```python
from build123d import *

# Parameters (mm, degrees)
F0_W      = 95.741764
F0_H      = 56.171074
F1_DEPTH  = 76.2
F1_FACE_W = 95.741764
F1_FACE_H = 56.171074
F2_DEPTH  = 25.4
F3_W      = 43.624266
F3_H      = 23.742414
F4_DEPTH  = 25.4


with BuildPart() as f1:
    # F0 (on Top) → F1 (new body)
    with BuildSketch(Plane.XY):
        Rectangle(F0_W, F0_H)
    extrude(amount=F1_DEPTH)

    # F1_face (on face) → F2 (join)
    with BuildSketch(Plane.XY.offset(76.2)):
        Rectangle(F1_FACE_W, F1_FACE_H)
    extrude(amount=F2_DEPTH)

    # F3 (on face) → F4 (cut)
    with BuildSketch(Plane.XY.offset(101.6)):
        Rectangle(F3_W, F3_H)
    extrude(amount=-F4_DEPTH, mode=Mode.SUBTRACT)


solid = f1.part
```
Model file for the job. Use its own axes, mm. A direction names the side the tool comes from. Coordinates: 2 decimals unless noted, no trailing zeros. Write each loop counter-clockwise with the first axis right and the second up, starting at its lowest first coordinate (ties: lowest second). Pieces come first, ordered by that corner, then holes. Notation, with made-up numbers: (3.25, 7) - (16.25, 7) arc R15 cw to (16.25, 20) - close; hole circle Ø1 at (25.5, 64.25). An arc over 180 degrees is marked (long way). One line per question, with ' | ' between items. Start each with the question number.
Q1. Pull direction X, two halves, no side cores. Call faces 3 (the face through (-47.871, 0, 50)), 4 (the face through (0, 11.871, 89)), 5 (the face through (0, 0, 76.2)), 6 (the face through (-1, 0, 0)): pulls with the +X half, pulls with the -X half, needs draft (parallel to the pull), parting line crosses it, or undercut.
Q2. Cut at B-B, the plane x = -10. List the corners of the cut face in (y, z), then the cut area to 3 significant figures.
Q3. Pin check, flat tip, straight feed: pin 1 (12 mm diameter, centred on x = 8, y = 5.5, fed in from +Z). Stop position of the tip, or through.
Q4. Cut at C-C, the plane y = -1. List the corners of the cut face in (x, z).
Q5. 3-axis set-ups, long thin cutter, end or side, ignore diameter. For faces 1 (the face through (-21.812, 0, 89)), 2 (the face through (47.871, 0, 50)): which of +Z, -Z, +X, -X, +Y, -Y reach the whole face in a straight line?
Q6. Cut at A-A, the plane z = 87.5. List the corners of the cut face in (x, y), then the cut area to 3 significant figures.
Q7. Drill centre lines: line 1 (Z direction, x = -5, y = 11); line 2 (Y direction, x = -2, z = 90). Where is each one in solid material? Low to high. Write a range as [from, to].
Answer below:
1) face 3: pulls with the -X half | face 4: undercut | face 5: undercut | face 6: needs draft
2) outline: (-28.09, 0) - (28.09, 0) - (28.09, 101.6) - (11.87, 101.6) - (11.87, 76.2) - (-11.87, 76.2) - (-11.87, 101.6) - (-28.09, 101.6) - close | area: 5,100 mm^2
3) pin 1: z = 76.2
4) outline: (-47.87, 0) - (47.87, 0) - (47.87, 101.6) - (21.81, 101.6) - (21.81, 76.2) - (-21.81, 76.2) - (-21.81, 101.6) - (-47.87, 101.6) - close
5) face 1: +Z | face 2: +Z, -Z, +X, +Y, -Y
6) outline: (-47.87, -28.09) - (47.87, -28.09) - (47.87, 28.09) - (-47.87, 28.09) - close; hole (-21.81, -11.87) - (21.81, -11.87) - (21.81, 11.87) - (-21.81, 11.87) - close | area: 4,340 mm^2
7) line 1: [0, 76.2] | line 2: [-28.09, -11.87], [11.87, 28.09]
